Geometry: final body of the model. Coordinates: model frame, mm. Coordinates: 2 decimals unless noted, no trailing zeros. Write each loop counter-clockwise with the first axis right and the second up, starting at its lowest first coordinate (ties: lowest second). Pieces come first, ordered by that corner, then holes. Notation, with made-up numbers: (-4.75, -30.75) - (16.25, -30.75) arc R18 cw to (16.25, -6.75) - close; hole circle Ø9 at (15.25, 43.5). An arc over 180 degrees is marked (long way). Put each result on its own line as item: value.
```python
from build123d import *

# Parameters (mm, degrees)
SKETCH1_R           = 6
BOSS_EXTRUDE1_DEPTH = 38
SKETCH3_R           = 6
CUT_EXTRUDE1_DEPTH  = 38


with BuildPart() as part:
    # Sketch1 → Boss-Extrude1 (new body)
    with BuildSketch(Plane(origin=(0, 0, 0), x_dir=(1, 0, 0), z_dir=(0, 1, 0))):
        with BuildLine():
            Line((0, 12.5), (50, 12.5))
            ThreePointArc((50, 12.5), (62.5, 0), (50, -12.5))
            Line((50, -12.5), (0, -12.5))
            ThreePointArc((0, -12.5), (-12.5, 0), (0, 12.5))
        make_face()
        Circle(SKETCH1_R, mode=Mode.SUBTRACT)
        with Locations((50, 0)):
            Circle(SKETCH1_R, mode=Mode.SUBTRACT)
    extrude(amount=BOSS_EXTRUDE1_DEPTH)

    # Sketch3 → Cut-Extrude1 (cut)
    with BuildSketch(Plane.XY.offset(12.5)):
        with Locations((25, 19)):
            Circle(SKETCH3_R)
    extrude(amount=-CUT_EXTRUDE1_DEPTH, mode=Mode.SUBTRACT)


solid = part.part
```
1. Pin query (flat end, axial travel): pin 1 Ø6 at (y, z) = (27, -7) entering from -X; pin 2 Ø9.5 at (x, z) = (50, 0) entering from +Y; pin 3 Ø1.5 at (x, y) = (-3.5, 19.5) entering from +Z; pin 4 Ø6 at (y, z) = (29, 5.5) entering from +X. Return the tip coordinate at first contact, or that it passes through.
Answer below:
pin 1: stops at x = -11.84
pin 2: passes through
pin 3: stops at z = 12.19
pin 4: stops at x = 62.25
2. Mould query, pull axis Y, two halves, no side actions, for faces 1 (the flat face through (19, 15, -12.5)), 2 (the cylindrical face through (19, 19, 0)), 3 (the flat face through (26, 0, 0)), 4 (the flat face through (26, 38, 0)). Classes: +Y half, -Y half, draft (parallel to the pull), parting line (faces both ways), or undercut.
Answer below:
face 1: draft
face 2: undercut
face 3: -Y half
face 4: +Y half
3. Section query A-A (z = 0). Return loops of the section in (x, y), then the cut area to 3 significant figures.
Answer below:
outline: (-12.5, 0) - (-6, 0) - (-6, 38) - (-12.5, 38) - close; (6, 0) - (44, 0) - (44, 38) - (6, 38) - close; (56, 0) - (62.5, 0) - (62.5, 38) - (56, 38) - close; hole circle Ø12 at (25, 19)
area: 1,820 mm²
4. Section query B-B (y = 19). Return loops of the section in (x, z), then the cut area to 3 significant figures.
Answer below:
outline: (0, -12.5) - (19, -12.5) - (19, 12.5) - (0, 12.5) arc R12.5 ccw to start; (31, -12.5) - (50, -12.5) arc R12.5 ccw to (50, 12.5) - (31, 12.5) - close; hole circle Ø12 at (0, 0); hole circle Ø12 at (50, 0)
area: 1,210 mm²
5. Section query C-C (x = 25). Return loops of the section in (y, z), then the cut area to 3 significant figures.
Answer below:
outline: (0, -12.5) - (13, -12.5) - (13, 12.5) - (0, 12.5) - close; (25, -12.5) - (38, -12.5) - (38, 12.5) - (25, 12.5) - close
area: 650 mm²
6. Section query D-D (y = 30). Return loops of the section in (x, z).
Answer below:
outline: (0, -12.5) - (50, -12.5) arc R12.5 ccw to (50, 12.5) - (0, 12.5) arc R12.5 ccw to start; hole circle Ø12 at (0, 0); hole circle Ø12 at (50, 0)
7. Ray query, probe 1 along X at (y, z) = (26, 0); probe 2 along Z at (x, y) = (0, 23.5); probe 3 along Y at (x, z) = (25, 5). Return the intervals inside material, ascending. Write a range as from..to.
Answer below:
probe 1: x = -12.5..-6, 6..44, 56..62.5
probe 2: z = -12.5..-6, 6..12.5
probe 3: y = 0..13, 25..38
